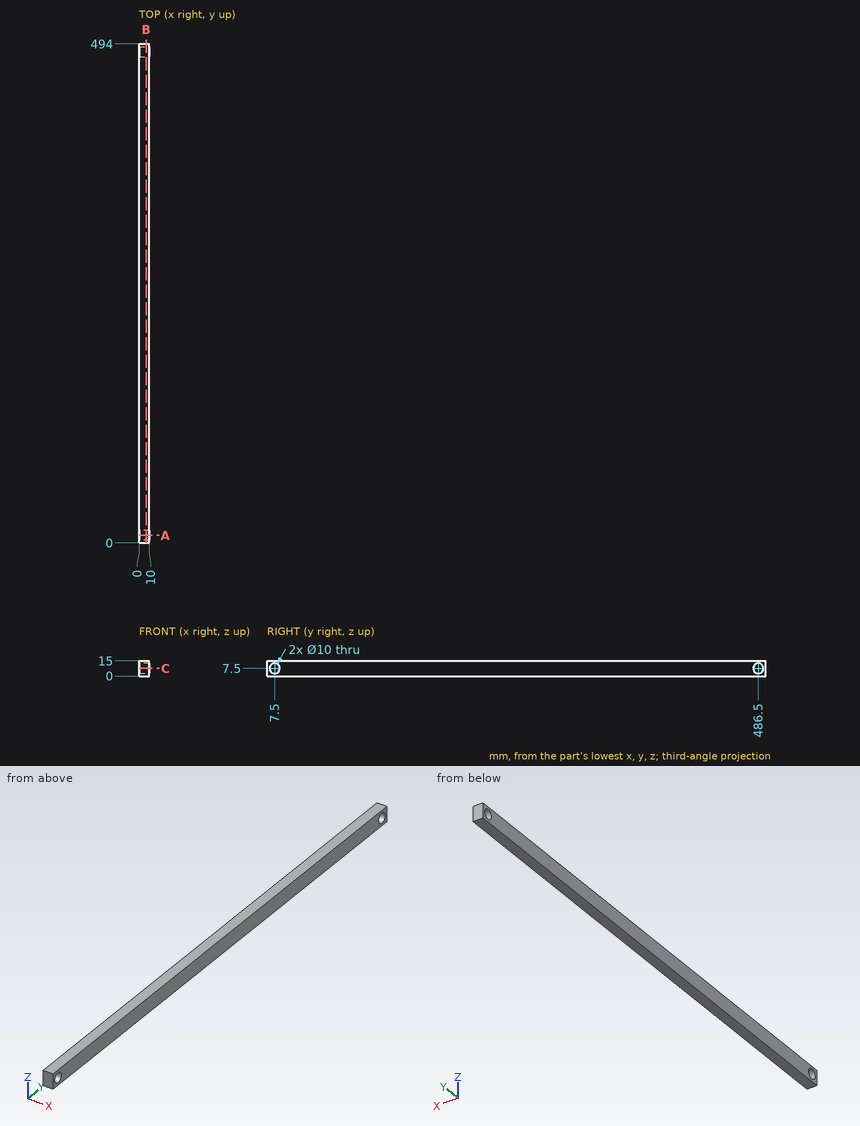
Check sheet for the drawn part. Datum: minimum x, y, z corner. Units: mm. Round coordinates to 2 decimals unless told otherwise and drop trailing zeros. Order: outer loops, then holes, each group sorted by start corner. A loop starts at its lowest first (then second) coordinate and runs counter-clockwise, first axis right, second up. Notation, with made-up numbers: (48, 26.5) -> (73, 26.5) arc R22 cw to (73, 64.5) -> close; hole circle Ø11 at (3, 2). An arc over 180 degrees is marked (long way). Put each result on its own line as item: value. Start each with the question number.
(1) Section check A-A (y = 7.5). Enter the section's corners in (x, z), then the cut area to 3 significant figures.
(2) Material ranges on line 1 along Y through (x, z) = (3.5, 7.5); line 2 along Z through (x, y) = (7.5, 486.5); line 3 along Y through (x, z) = (1.75, 11), recorded low to high.
(3) Depth check by flat-ended pin: pin 1 Ø1.5 at (y, z) = (125.5, 13) entering from -X. Enter the tip coordinate at first touch or a pass-through.
(4) Section check B-B (x = 7). Enter the section's corners in (y, z).
(5) Section check C-C (z = 7.5). Enter the section's corners in (x, y).
Completed:
1. outline: (0, 0) -> (10, 0) -> (10, 2.5) -> (0, 2.5) -> close; (0, 12.5) -> (10, 12.5) -> (10, 15) -> (0, 15) -> close
1. area: 50.0 mm2
2. line 1: y = 0 to 2.5, 12.5 to 481.5, 491.5 to 494
2. line 2: z = 0 to 2.5, 12.5 to 15
2. line 3: y = 0 to 3.93, 11.07 to 482.93, 490.07 to 494
3. pin 1: stops at x = 0
4. outline: (0, 0) -> (494, 0) -> (494, 15) -> (0, 15) -> close; hole circle Ø10 at (7.5, 7.5); hole circle Ø10 at (486.5, 7.5)
5. outline: (0, 0) -> (10, 0) -> (10, 2.5) -> (0, 2.5) -> close; (0, 12.5) -> (10, 12.5) -> (10, 481.5) -> (0, 481.5) -> close; (0, 491.5) -> (10, 491.5) -> (10, 494) -> (0, 494) -> close
